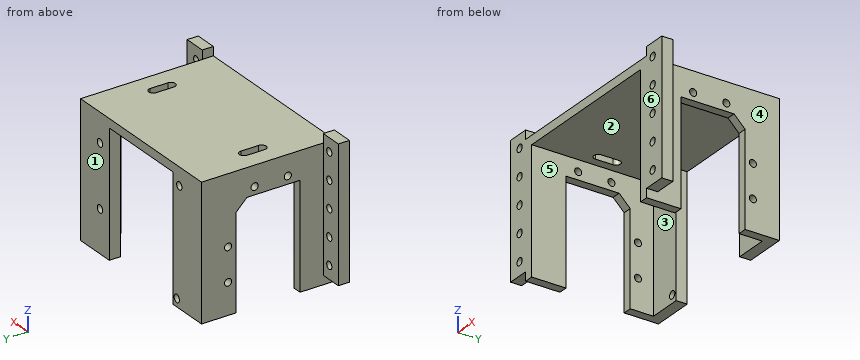
from build123d import *

# Parameters (mm, degrees)
SKETCH_1_W           = 80
SKETCH_1_H           = 60
EXTRUDE_1_DEPTH      = 30
SKETCH_2_W           = 72
SKETCH_2_H           = 56
CUT_EXTRUDE_1_DEPTH  = 70
SKETCH_3_W           = 47.385697094
SKETCH_3_H           = 29
CUT_EXTRUDE_2_DEPTH  = 80
SKETCH_4_W           = 10
SKETCH_4_H           = 60
EXTRUDE_2_DEPTH      = 5
SKETCH_5_R           = 1.7
CUT_EXTRUDE_3_DEPTH  = 25
SKETCH_6_W           = 15
SKETCH_6_H           = 56
EXTRUDE_3_DEPTH      = 5
SKETCH_8_R           = 1.75
CUT_EXTRUDE_5_DEPTH  = 10
CHAMFER_1_SIZE       = 5
CUT_EXTRUDE_8_DEPTH  = 10
SKETCH_11_R          = 1.6
CUT_EXTRUDE_9_DEPTH  = 100
SKETCH_12_R          = 1.6
CUT_EXTRUDE_10_DEPTH = 120


with BuildPart() as part:
    # 草图1 → 凸台-拉伸1 (new, symmetric)
    with BuildSketch(Plane(origin=(0, 0, 0), x_dir=(1, 0, 0), z_dir=(0, 1, 0))):
        Rectangle(SKETCH_1_W, SKETCH_1_H)
    extrude(amount=EXTRUDE_1_DEPTH, both=True)

    # 草图2 → 切除-拉伸1 (cut)
    with BuildSketch(Plane(origin=(0, 30, 0), x_dir=(1, 0, 0), z_dir=(0, 1, 0))):
        with Locations((0, 2)):
            Rectangle(SKETCH_2_W, SKETCH_2_H)
    extrude(amount=-CUT_EXTRUDE_1_DEPTH, mode=Mode.SUBTRACT)

    # 草图3 → 切除-拉伸2 (cut)
    with BuildSketch(Plane(origin=(40, 0, 0), x_dir=(0, 0, -1), z_dir=(1, 0, 0))):
        with Locations((6.307151453, 0)):
            Rectangle(SKETCH_3_W, SKETCH_3_H)
    extrude(amount=-CUT_EXTRUDE_2_DEPTH, mode=Mode.SUBTRACT)

    # 草图4 → 凸台-拉伸2 (add)
    with BuildSketch(Plane.XZ.offset(30)):
        with Locations((-45, 4)):
            Rectangle(SKETCH_4_W, SKETCH_4_H)
        with Locations((45, 4)):
            Rectangle(SKETCH_4_W, SKETCH_4_H)
    extrude(amount=-EXTRUDE_2_DEPTH)

    # 草图5 → 切除-拉伸3 (cut)
    with BuildSketch(Plane(origin=(0, -25, 0), x_dir=(1, 0, 0), z_dir=(0, 1, 0))):
        with Locations(Location((-44, 20, 0), (0, 0, 270))):
            Circle(SKETCH_5_R)
        with Locations(Location((-44, 8, 0), (0, 0, 270))):
            Circle(SKETCH_5_R)
        with Locations(Location((-44, -4, 0), (0, 0, 270))):
            Circle(SKETCH_5_R)
        with Locations(Location((-44, -16, 0), (0, 0, 270))):
            Circle(SKETCH_5_R)
        with Locations(Location((-44, -28, 0), (0, 0, 270))):
            Circle(SKETCH_5_R)
        with Locations(Location((44, -28, 0), (0, 0, 90))):
            Circle(SKETCH_5_R)
        with Locations(Location((44, -16, 0), (0, 0, 90))):
            Circle(SKETCH_5_R)
        with Locations(Location((44, -4, 0), (0, 0, 90))):
            Circle(SKETCH_5_R)
        with Locations(Location((44, 8, 0), (0, 0, 90))):
            Circle(SKETCH_5_R)
        with Locations(Location((44, 20, 0), (0, 0, 90))):
            Circle(SKETCH_5_R)
    extrude(amount=-CUT_EXTRUDE_3_DEPTH, mode=Mode.SUBTRACT)

    # 草图6 → 凸台-拉伸3 (add)
    with BuildSketch(Plane(origin=(0, 30, 0), x_dir=(1, 0, 0), z_dir=(0, 1, 0))):
        with Locations((-28.5, 2)):
            Rectangle(SKETCH_6_W, SKETCH_6_H)
        with Locations((28.5, 2)):
            Rectangle(SKETCH_6_W, SKETCH_6_H)
    extrude(amount=-EXTRUDE_3_DEPTH)

    # 草图8 → 切除-拉伸5 (cut)
    with BuildSketch(Plane(origin=(0, 30, 0), x_dir=(1, 0, 0), z_dir=(0, 1, 0))):
        with Locations(Location((-25.32, -22, 0), (0, 0, 270))):
            Circle(SKETCH_8_R)
        with Locations(Location((-23.61, 26.395, 0), (0, 0, 270))):
            Circle(SKETCH_8_R)
        with Locations(Location((27.2, 10.96, 0), (0, 0, 270))):
            Circle(SKETCH_8_R)
        with Locations(Location((27.2, -17, 0), (0, 0, 270))):
            Circle(SKETCH_8_R)
    extrude(amount=-CUT_EXTRUDE_5_DEPTH, mode=Mode.SUBTRACT)

    # 倒角1
    chamfer_1_edges = [part.edges().sort_by_distance(p)[0] for p in [
        (38, 14.5, 17.385697094),
        (-38, 14.5, 17.385697094),
    ]]
    chamfer(chamfer_1_edges, length=CHAMFER_1_SIZE)

    # 草图10 → 切除-拉伸8 (cut)
    with BuildSketch(Plane.XY.offset(30)):
        with BuildLine():
            Line((-28, 4), (-28, -4))
            ThreePointArc((-28, -4), (-30, -6), (-32, -4))
            Line((-32, -4), (-32, 4))
            ThreePointArc((-32, 4), (-30, 6), (-28, 4))
        make_face()
        with BuildLine():
            Line((28, 4), (28, -4))
            ThreePointArc((28, -4), (30, -6), (32, -4))
            Line((32, -4), (32, 4))
            ThreePointArc((32, 4), (30, 6), (28, 4))
        make_face()
    extrude(amount=-CUT_EXTRUDE_8_DEPTH, mode=Mode.SUBTRACT)

    # 草图11 → 切除-拉伸9 (cut)
    with BuildSketch(Plane.ZY.offset(40)):
        with Locations((-16, 18)):
            Circle(SKETCH_11_R)
        with Locations((-1, 18)):
            Circle(SKETCH_11_R)
    extrude(amount=-CUT_EXTRUDE_9_DEPTH, mode=Mode.SUBTRACT)

    # 草图12 → 切除-拉伸10 (cut)
    with BuildSketch(Plane.ZY.offset(40)):
        with Locations((20.885697094, 6)):
            Circle(SKETCH_12_R)
        with Locations((20.885697094, -9)):
            Circle(SKETCH_12_R)
    extrude(amount=-CUT_EXTRUDE_10_DEPTH, mode=Mode.SUBTRACT)


solid = part.part
Read the model definition and answer for the solid it produces. Units are mm, in the model's axes. Face numbers are marked on the shaded views. A direction names the side the tool comes from. Coordinates: 2 decimals unless noted, no trailing zeros. Write each loop counter-clockwise with the first axis right and the second up, starting at its lowest first coordinate (ties: lowest second). Pieces come first, ordered by that corner, then holes. Notation, with made-up numbers: (-39, 50) -> (-27, 50) arc R25 ccw to (-27, 72) -> close; hole circle Ø11 at (38, 20.5). An arc over 180 degrees is marked (long way). Return JSON: item names as keys, results as strings.
(1) The part is cut by section D-D on x = 24. Give the vertices of the cut face in (y, z), then the cut area to 3 significant figures.
Answers below:
{"outline": "(-30, 26) -> (25, 26) -> (25, -30) -> (30, -30) -> (30, 30) -> (-30, 30) -> close", "area": "520 mm^2"}
(2) For a pull along X with two mould halves and no side action, classify the marked faces 3, 4, 5 and 6 as pulls with the +X half, pulls with the -X half, needs draft (parallel to the pull), parting line crosses it, or undercut.
Answers below:
{"face 3": "undercut", "face 4": "pulls with the +X half", "face 5": "undercut", "face 6": "needs draft"}
(3) The part is cut by section B-B on z = 11. Give the vertices of the cut face in (x, y).
Answers below:
{"outline": "(-50, -30) -> (-36, -30) -> (-36, -14.5) -> (-40, -14.5) -> (-40, -25) -> (-50, -25) -> close; (-40, 14.5) -> (-36, 14.5) -> (-36, 25) -> (-21, 25) -> (-21, 30) -> (-40, 30) -> close; (21, 25) -> (36, 25) -> (36, 14.5) -> (40, 14.5) -> (40, 30) -> (21, 30) -> close; (36, -30) -> (50, -30) -> (50, -25) -> (40, -25) -> (40, -14.5) -> (36, -14.5) -> close"}
(4) The part is cut by section C-C on y = -23. Give the vertices of the cut face in (x, z), then the cut area to 3 significant figures.
Answers below:
{"outline": "(-40, -30) -> (-36, -30) -> (-36, 26) -> (36, 26) -> (36, -30) -> (40, -30) -> (40, 30) -> (-40, 30) -> close", "area": "768 mm^2"}
(5) Which of the six approach directions +Z, -Z, +X, -X, +Y, -Y give full straight-line access (tool end or side, diameter ignored) to the marked faces 1 and 2?
Answers below:
{"face 1": "+Z, -Z, +X, -X, +Y", "face 2": "-Z, -Y"}
(6) Consider line 1 along X through (y, z) = (-28, 28); line 2 along Z through (x, y) = (44, -28.8); line 3 along X through (y, z) = (26.6, -10.96). Determine where each line is inside the solid, lowest interval first. Write a range as from..to.
Answers below:
{"line 1": "-50..-45.7, -42.3..42.3, 45.7..50", "line 2": "-26..-21.7, -18.3..-9.7, -6.3..2.3, 5.7..14.3, 17.7..26.3, 29.7..34", "line 3": "-40..-21, 21..25.45, 28.95..40"}
(7) Each of these flat-tipped pins is pushed along its axis until it touches: P1, Ø2.5, axis at y = -9, z = 20.89, coming from the +X side; P2, Ø1.2, axis at y = -1.5, z = 27, coming from the +X side; P3, Ø7.5, axis at x = -28.5, z = 12, coming from the -Y side; P4, Ø18, axis at x = 9, y = -5, coming from the +Z side. Where does it stop, or does it pass through?
Answers below:
{"P1": "through", "P2": "x = 40", "P3": "y = 25", "P4": "z = 30"}
(8) The part is cut by section A-A on z = 4. State how many separate pieces and enclosed holes the cut face has, then the cut area to 3 significant figures.
Answers below:
{"separate pieces": "6", "enclosed holes": "0", "area": "464 mm^2"}
